Design review of the part built by this model. Coordinates are the model's own, in mm. A direction names the side the tool comes from. Coordinates: 2 decimals unless noted, no trailing zeros. Loops run counter-clockwise (first coordinate to the right, second up) from the corner with the lowest first, then second, coordinate; pieces in that order, holes last.
Q1. Add section A-A on y = 30.5. Give the boundary of the cut face in (x, z), and give its area (3 significant figures).
Q2. For P1, Ø1, axis at x = 43.5, z = -22, coming from the -Y side; P2, Ø2.5, axis at x = 35.5, z = 20, coming from the +Y side; P3, Ø6, axis at x = 28, z = -43, coming from the -Y side, all flat-tipped, find the tip position at first contact; note any pin that passes through.
Q3. Draft analysis for pull direction X (two halves, no side actions). For faces 1 (the face through (0, 3, -22)), 2 (the face through (33, -4, -62)), 3 (the face through (36, -1.5, -66)), 4 (the face through (51, -4, -22)), state which applies: released by +X, released by -X, zero draft, split by the parting line, or undercut.
Q4. Add section C-C on y = 12. Give the boundary of the cut face in (x, z), and give its area (3 significant figures).
Q5. Add section B-B on z = -22.5. Give the boundary of the cut face in (x, y), and give its area (3 significant figures).
Q6. Machinability: for faces 5 (the face through (22.815, 7.203, -1.141)), 6 (the face through (45, 15, 12)), 7 (the face through (35.5, -6.85, 27.99)), which of the approach directions +Z, -Z, +X, -X, +Y, -Y give a long, thin tool a straight path to every point of the face, cutting with its end or side? Answer none if there is none.
Q7. Wall thickness on probe 1 along X at (y, z) = (2.7, -7); probe 2 along Z at (x, y) = (36.5, -21.5); probe 3 along Z at (x, y) = (37, 2): over which ranges is each line inside the solid? List them lowest first.
```python
from build123d import *
from OCP.BRepFilletAPI import BRepFilletAPI_MakeFillet

# Parameters (mm, degrees)
SKETCH2_W                  = 45
SKETCH2_H                  = 45
BOSS_EXTRUDE1_DEPTH        = 6
SKETCH4_R                  = 11.5
SKETCH4_R_2                = 2
CUT_EXTRUDE1_DEPTH         = 64.921827258
SKETCH5_W                  = 6
SKETCH5_H                  = 45
BOSS_EXTRUDE2_DEPTH        = 30.1
BOSS_EXTRUDE2_DEPTH_BACK   = 36
BOSS_EXTRUDE3_DEPTH        = 3
BOSS_EXTRUDE4_DEPTH        = 3
BOSS_EXTRUDE5_DEPTH        = 28
BOSS_EXTRUDE6_DEPTH        = 5
FILLET3_R                  = 10
FILLET4_R1                 = 4
FILLET4_R2                 = 2
FILLET4_R3                 = 1.2
FILLET4_R4                 = 1.5
BOSS_EXTRUDE7_DEPTH        = 28
BOSS_EXTRUDE8_DEPTH        = 5
FILLET5_R                  = 10
F_6_5_6_5_DIAMETER_HOLE1_D = 6.5
SKETCH14_R                 = 4
CUT_EXTRUDE2_DEPTH         = 7.5
BOSS_EXTRUDE9_DEPTH        = 6


with BuildPart() as part:
    # Sketch2 → Boss-Extrude1 (new body)
    with BuildSketch(Plane(origin=(0, 0, 0), x_dir=(1, 0, 0), z_dir=(0, 1, 0))):
        with Locations((22.5, 22.5)):
            Rectangle(SKETCH2_W, SKETCH2_H)
    extrude(amount=BOSS_EXTRUDE1_DEPTH)

    # Sketch4 → Cut-Extrude1 (cut, through all)
    with BuildSketch(Plane(origin=(0, 6, 0), x_dir=(-1, 0, 0), z_dir=(0, 1, 0))):
        with Locations(Location((-22, -22.5, 0), (0, 0, 90))):
            Circle(SKETCH4_R)
        with Locations(Location((-37.5, -7, 0), (0, 0, 90))):
            Circle(SKETCH4_R_2)
        with Locations(Location((-6.5, -7, 0), (0, 0, 90))):
            Circle(SKETCH4_R_2)
        with Locations(Location((-6.5, -38, 0), (0, 0, 90))):
            Circle(SKETCH4_R_2)
        with Locations(Location((-37.5, -38, 0), (0, 0, 90))):
            Circle(SKETCH4_R_2)
    extrude(amount=-CUT_EXTRUDE1_DEPTH, mode=Mode.SUBTRACT)

    # Sketch5 → Boss-Extrude2 (add, two sides)
    with BuildSketch(Plane.XZ) as boss_extrude2_sk:
        with Locations((48, -22.5)):
            Rectangle(SKETCH5_W, SKETCH5_H)
    extrude(amount=BOSS_EXTRUDE2_DEPTH)
    extrude(boss_extrude2_sk.sketch, amount=-BOSS_EXTRUDE2_DEPTH_BACK)

    # Sketch8 → Boss-Extrude3 (add)
    with BuildSketch(Plane.XY):
        Polygon((45, 36), (0, 6), (0, 0), (45, -30.1), (51, -30.1), (51, 36), align=None)
    extrude(amount=BOSS_EXTRUDE3_DEPTH)

    # Sketch9 → Boss-Extrude4 (add)
    with BuildSketch(Plane(origin=(0, 0, -45), x_dir=(-1, 0, 0), z_dir=(0, 0, -1))):
        Polygon((0, 6), (-45, 36), (-51, 36), (-51, -30.1), (-45, -30.1), (0, 0), align=None)
    extrude(amount=BOSS_EXTRUDE4_DEPTH)

    # Sketch11 → Boss-Extrude5 (add)
    with BuildSketch(Plane.XY.offset(3)):
        Polygon((51, -30.1), (45, -30.1), (45, -4), (21, -4), (21, 6), (51, 6), align=None)
    extrude(amount=BOSS_EXTRUDE5_DEPTH)

    # Sketch12 → Boss-Extrude6 (add)
    with BuildSketch(Plane.XY.offset(31)):
        Polygon((45, -30.1), (21, -4), (21, 6), (51, 6), (51, -30.1), align=None)
    extrude(amount=BOSS_EXTRUDE6_DEPTH)

    # Fillet3
    fillet3_edges = [part.edges().sort_by_distance(p)[0] for p in [
        (33, -4, 3),
        (33, -4, 31),
    ]]
    fillet(fillet3_edges, radius=FILLET3_R)

    # Fillet4: one fillet with a radius per group of edges: ONE call of the kernel's fillet builder (fillet() takes one radius for all edges)
    fillet4_edges_1 = [part.edges().sort_by_distance(p)[0] for p in [
        (22.5, 6, -45),
        (22.5, 6, 0),
    ]]
    fillet4_edges_2 = [part.edges().sort_by_distance(p)[0] for p in [
        (45, 6, -22.5),
    ]]
    fillet4_edges_3 = [part.edges().sort_by_distance(p)[0] for p in [
        (22.5, 0, -45),
        (22.5, 0, 0),
    ]]
    fillet4_edges_4 = [part.edges().sort_by_distance(p)[0] for p in [
        (45, 0, -22.5),
    ]]
    fillet4 = BRepFilletAPI_MakeFillet(part.part.solid().wrapped)
    for e in fillet4_edges_1:
        fillet4.Add(FILLET4_R1, e.wrapped)
    for e in fillet4_edges_2:
        fillet4.Add(FILLET4_R2, e.wrapped)
    for e in fillet4_edges_3:
        fillet4.Add(FILLET4_R3, e.wrapped)
    for e in fillet4_edges_4:
        fillet4.Add(FILLET4_R4, e.wrapped)
    add(Compound.cast(fillet4.Shape()), mode=Mode.REPLACE)

    # Sketch15 → Boss-Extrude7 (add)
    with BuildSketch(Plane(origin=(0, 0, -48), x_dir=(-1, 0, 0), z_dir=(0, 0, -1))):
        Polygon((-51, -30.1), (-51, 6), (-21, 6), (-21, -4), (-45, -4), (-45, -30.1), align=None)
    extrude(amount=BOSS_EXTRUDE7_DEPTH)

    # Sketch16 → Boss-Extrude8 (add)
    with BuildSketch(Plane(origin=(0, 0, -76), x_dir=(-1, 0, 0), z_dir=(0, 0, -1))):
        Polygon((-45, -30.1), (-21, -4), (-21, 6), (-51, 6), (-51, -30.1), align=None)
    extrude(amount=BOSS_EXTRUDE8_DEPTH)

    # Fillet5
    fillet5_edges = [part.edges().sort_by_distance(p)[0] for p in [
        (33, -4, -48),
        (33, -4, -76),
    ]]
    fillet(fillet5_edges, radius=FILLET5_R)

    # 6.5 _6.5_ Diameter Hole1 (through all)
    with Locations(Plane.ZY.offset(-45)):
        with Locations((-22.5, 12), (-22.5, 30.5), (-37, -15), (-8, -15), (21, -15), (-66, -15)):
            Hole(F_6_5_6_5_DIAMETER_HOLE1_D / 2)

    # Sketch14 → Cut-Extrude2 (cut)
    with BuildSketch(Plane(origin=(0, 6, 0), x_dir=(1, 0, 0), z_dir=(0, 1, 0))):
        with Locations(Location((36, -21, 0), (0, 0, 180))):
            Circle(SKETCH14_R)
        with Locations(Location((36, 66, 0), (0, 0, 180))):
            Circle(SKETCH14_R)
    extrude(amount=-CUT_EXTRUDE2_DEPTH, mode=Mode.SUBTRACT)

    # Sketch17 → Boss-Extrude9 (add)
    with BuildSketch(Plane(origin=(51, 0, 0), x_dir=(0, 0, -1), z_dir=(1, 0, 0))):
        Polygon((-3, 36), (-36, 6), (-3, 6), align=None)
        Polygon((48, 36), (81, 6), (48, 6), align=None)
    extrude(amount=-BOSS_EXTRUDE9_DEPTH)


solid = part.part
```
Entries:
1. outline: (36.75, -48) - (45, -48) - (45, -54.05) - (51, -54.05) - (51, -25.75) - (45, -25.75) - (45, -45) - (36.75, -45) - close; (36.75, 0) - (45, 0) - (45, -19.25) - (51, -19.25) - (51, 9.05) - (45, 9.05) - (45, 3) - (36.75, 3) - close
1. area: 389 mm2
2. P1: stops at y = -0.09
2. P2: stops at y = -1.5
2. P3: stops at y = -20.22
3. face 1: released by -X
3. face 2: zero draft
3. face 3: undercut
3. face 4: released by +X
4. outline: (9, -48) - (45, -48) - (45, -74.4) - (51, -74.4) - (51, -25.75) - (45, -25.75) - (45, -45) - (9, -45) - close; (9, 0) - (45, 0) - (45, -19.25) - (51, -19.25) - (51, 29.4) - (45, 29.4) - (45, 3) - (9, 3) - close
4. area: 800 mm2
5. outline: (0, 0) - (10.5, 0) - (10.5, 6) - (0, 6) - close; (33.5, 0) - (43.5, 0) arc R1.5 cw to (45, -1.5) - (45, -30.1) - (51, -30.1) - (51, 8.75) - (45, 8.75) - (45, 8) arc R2 cw to (43, 6) - (33.5, 6) - close; (45, 15.25) - (51, 15.25) - (51, 27.25) - (45, 27.25) - close; (45, 33.75) - (51, 33.75) - (51, 36) - (45, 36) - close
5. area: 452 mm2
6. face 5: -X, +Y
6. face 6: +Z, -X, +Y
6. face 7: -X, -Y
7. probe 1: x = 0 to 4.5, 8.5 to 35.5, 39.5 to 51
7. probe 2: z = -48 to -45, 0 to 3
7. probe 3: z = -81 to -69.87, -62.13 to -39.94, -36.06 to -8.94, -5.06 to 17.13, 24.87 to 36
